```python
from build123d import *

# Parameters (mm, degrees)
SKETCH1_W           = 224
SKETCH1_H           = 24
BOSS_EXTRUDE1_DEPTH = 8
SKETCH2_R           = 2.05
CUT_EXTRUDE1_DEPTH  = 9
SKETCH3_W           = 4
SKETCH3_H           = 6.5
CUT_EXTRUDE2_DEPTH  = 225


with BuildPart() as part:
    # Sketch1 → Boss-Extrude1 (new body)
    with BuildSketch(Plane(origin=(0, 0, 0), x_dir=(1, 0, 0), z_dir=(0, 1, 0))):
        Rectangle(SKETCH1_W, SKETCH1_H)
    extrude(amount=BOSS_EXTRUDE1_DEPTH)

    # Sketch2 → Cut-Extrude1 (cut, through all)
    with BuildSketch(Plane(origin=(0, 8, 0), x_dir=(1, 0, 0), z_dir=(0, 1, 0))):
        with Locations((-104, 8)):
            Circle(SKETCH2_R)
        with Locations((-88, 8)):
            Circle(SKETCH2_R)
        with Locations((-72, 8)):
            Circle(SKETCH2_R)
        with Locations((-56, 8)):
            Circle(SKETCH2_R)
        with Locations((-40, 8)):
            Circle(SKETCH2_R)
        with Locations((-24, 8)):
            Circle(SKETCH2_R)
        with Locations((-8, 8)):
            Circle(SKETCH2_R)
        with Locations((8, 8)):
            Circle(SKETCH2_R)
        with Locations((24, 8)):
            Circle(SKETCH2_R)
        with Locations((40, 8)):
            Circle(SKETCH2_R)
        with Locations((56, 8)):
            Circle(SKETCH2_R)
        with Locations((72, 8)):
            Circle(SKETCH2_R)
        with Locations((88, 8)):
            Circle(SKETCH2_R)
        with Locations((104, 8)):
            Circle(SKETCH2_R)
        with Locations((-88, -8)):
            Circle(SKETCH2_R)
        with Locations((-72, -8)):
            Circle(SKETCH2_R)
        with Locations((-56, -8)):
            Circle(SKETCH2_R)
        with Locations((-40, -8)):
            Circle(SKETCH2_R)
        with Locations((-24, -8)):
            Circle(SKETCH2_R)
        with Locations((-8, -8)):
            Circle(SKETCH2_R)
        with Locations((8, -8)):
            Circle(SKETCH2_R)
        with Locations((24, -8)):
            Circle(SKETCH2_R)
        with Locations((40, -8)):
            Circle(SKETCH2_R)
        with Locations((56, -8)):
            Circle(SKETCH2_R)
        with Locations((72, -8)):
            Circle(SKETCH2_R)
        with Locations((88, -8)):
            Circle(SKETCH2_R)
        with Locations((104, -8)):
            Circle(SKETCH2_R)
        with Locations((-104, -8)):
            Circle(SKETCH2_R)
    extrude(amount=-CUT_EXTRUDE1_DEPTH, mode=Mode.SUBTRACT)

    # Sketch3 → Cut-Extrude2 (cut, through all)
    with BuildSketch(Plane.ZY.offset(112)):
        with Locations((0, 4.75)):
            Rectangle(SKETCH3_W, SKETCH3_H)
        Polygon((-12, 6.85), (-10.65, 5.5), (-10.65, 2.5), (-12, 1.15), align=None)
        Polygon((12, 6.85), (12, 1.15), (10.65, 2.5), (10.65, 5.5), align=None)
    extrude(amount=-CUT_EXTRUDE2_DEPTH, mode=Mode.SUBTRACT)


solid = part.part
```
CAD build for the part. Positions are in the model's coordinates, mm. A direction names the side the tool comes from. Round coordinates to 2 decimals unless told otherwise and drop trailing zeros. Order: outer loops, then holes, each group sorted by start corner. A loop starts at its lowest first (then second) coordinate and runs counter-clockwise, first axis right, second up.
Q1. Which spindle directions (+Z, -Z, +X, -X, +Y, -Y) get a long thin tool onto all of the face, cutting with end or side? Do faces 3 (the cylindrical face through (-58.05, 4.06, 7.91)), 4 (the flat face through (-2, 5, -2)). Say none if no direction does.
Q2. Wall check: L1, parallel to Z at x = 8, y = 5; L2, parallel to Z at x = 20, y = 5.5; L3, parallel to Z at x = 54.5, y = 1.75. Give the ranges that are in metal, low to high.
Q3. Two-plate mould, pull along Z, no slides. Class faces 1 (the cylindrical face through (5.95, 4.06, -8.09)), 2 (the flat face through (-2, 0, 0)): pulls with the +Z half, pulls with the -Z half, needs draft (parallel to the pull), parting line crosses it, or undercut.
Q4. Slice it at B-B (x = -1). Write the cut outline in (y, z), and give its area (3 significant figures).
Q5. Drop flat-ended pins along their axis: pin 1 (1 mm diameter, centred on x = 23.5, y = 4.5, fed in from -Z); pin 2 (2.5 mm diameter, centred on x = 54, y = 4, fed in from +Z). Give the stop position or say it passes through.
Q6. Slice it at A-A (x = -56). Write the cut outline in (y, z).
Results below:
1. face 3: +Y, -Y
1. face 4: +X, -X, +Y
2. L1: z = -10.65 to -10.05, -5.95 to -2, 2 to 5.95, 10.05 to 10.65
2. L2: z = -10.65 to -2, 2 to 10.65
2. L3: z = -11.4 to -9.4, -6.6 to -2, 2 to 6.6, 9.4 to 11.4
3. face 1: undercut
3. face 2: needs draft
4. outline: (0, -12) - (1.15, -12) - (2.5, -10.65) - (5.5, -10.65) - (6.85, -12) - (8, -12) - (8, -2) - (1.5, -2) - (1.5, 2) - (8, 2) - (8, 12) - (6.85, 12) - (5.5, 10.65) - (2.5, 10.65) - (1.15, 12) - (0, 12) - close
4. area: 154 mm2
5. pin 1: stops at z = -10.65
5. pin 2: stops at z = 10.65
6. outline: (0, -12) - (1.15, -12) - (2.5, -10.65) - (5.5, -10.65) - (6.85, -12) - (8, -12) - (8, -10.05) - (0, -10.05) - close; (0, -5.95) - (8, -5.95) - (8, -2) - (1.5, -2) - (1.5, 2) - (8, 2) - (8, 5.95) - (0, 5.95) - close; (0, 10.05) - (8, 10.05) - (8, 12) - (6.85, 12) - (5.5, 10.65) - (2.5, 10.65) - (1.15, 12) - (0, 12) - close
